```python
from build123d import *

# Parameters (mm, degrees)
SKETCH1_W           = 234
SKETCH1_H           = 75
BOSS_EXTRUDE1_DEPTH = 5.7
SKETCH2_W           = 5.7
SKETCH2_H           = 55
CUT_EXTRUDE1_DEPTH  = 5.7
SKETCH3_W           = 174
SKETCH3_H           = 5.7
CUT_EXTRUDE2_DEPTH  = 5.7
SKETCH4_R           = 1.5
CUT_EXTRUDE3_DEPTH  = 2


with BuildPart() as part:
    # Sketch1 → Boss-Extrude1 (new body)
    with BuildSketch(Plane(origin=(0, 0, 0), x_dir=(1, 0, 0), z_dir=(0, 1, 0))):
        with Locations((117, 37.5)):
            Rectangle(SKETCH1_W, SKETCH1_H)
    extrude(amount=BOSS_EXTRUDE1_DEPTH)

    # Sketch2 → Cut-Extrude1 (cut)
    with BuildSketch(Plane(origin=(0, 5.7, 0), x_dir=(1, 0, 0), z_dir=(0, 1, 0))):
        with Locations((2.85, 37.5)):
            Rectangle(SKETCH2_W, SKETCH2_H)
        with Locations((231.15, 37.5)):
            Rectangle(SKETCH2_W, SKETCH2_H)
    extrude(amount=-CUT_EXTRUDE1_DEPTH, mode=Mode.SUBTRACT)

    # Sketch3 → Cut-Extrude2 (cut)
    with BuildSketch(Plane(origin=(0, 5.7, 0), x_dir=(1, 0, 0), z_dir=(0, 1, 0))):
        with Locations((117, 2.85)):
            Rectangle(SKETCH3_W, SKETCH3_H)
    extrude(amount=-CUT_EXTRUDE2_DEPTH, mode=Mode.SUBTRACT)

    # Sketch4 → Cut-Extrude3 (cut)
    with BuildSketch(Plane(origin=(0, 5.7, 0), x_dir=(1, 0, 0), z_dir=(0, 1, 0))):
        with Locations(Location((213.3, 45.7, 0), (0, 0, 270))):
            Circle(SKETCH4_R)
        with Locations(Location((213.3, 10.7, 0), (0, 0, 270))):
            Circle(SKETCH4_R)
        with Locations(Location((20.7, 10.7, 0), (0, 0, 270))):
            Circle(SKETCH4_R)
        with Locations(Location((20.7, 45.7, 0), (0, 0, 270))):
            Circle(SKETCH4_R)
    extrude(amount=-CUT_EXTRUDE3_DEPTH, mode=Mode.SUBTRACT)


solid = part.part
```
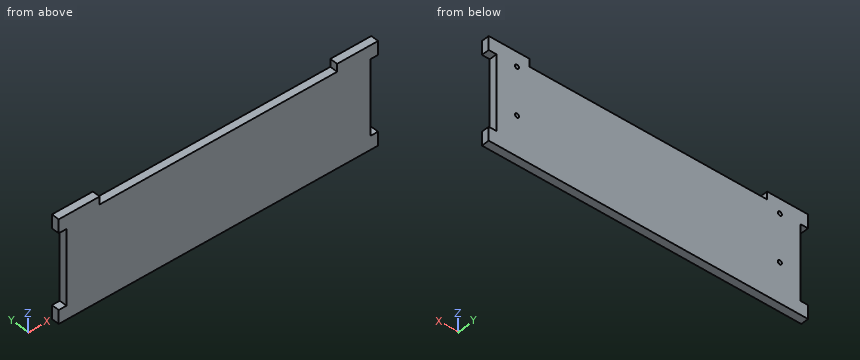
Geometry check sheet. Reference: the model listing, model coordinates, mm. Coordinates: 2 decimals unless noted, no trailing zeros. Write each loop counter-clockwise with the first axis right and the second up, starting at its lowest first coordinate (ties: lowest second). Pieces come first, ordered by that corner, then holes. Notation, with made-up numbers: M 35.5,-30 L 66.5,-30 A18 cw 66.5,-9 Z; hole C -26,69 d6. An arc over 180 degrees is marked long. Answer as a JSON object with one key per item and string values.
1. Section check A-A, the plane y = 2.2. Enter the section's corners in (x, z).
Answers below:
{"outline": "M 0,-75 L 234,-75 L 234,-65 L 228.3,-65 L 228.3,-10 L 234,-10 L 234,0 L 204,0 L 204,-5.7 L 30,-5.7 L 30,0 L 0,0 L 0,-10 L 5.7,-10 L 5.7,-65 L 0,-65 Z"}
2. Section check C-C, the plane z = -35.5. Enter the section's corners in (x, y), plus the area to 3 significant figures.
Answers below:
{"outline": "M 5.7,0 L 228.3,0 L 228.3,5.7 L 5.7,5.7 Z", "area": "1,270 mm²"}
3. Section check B-B, the plane x = 96.5. Enter the section's corners in (y, z), plus the area to 3 significant figures.
Answers below:
{"outline": "M 0,-75 L 5.7,-75 L 5.7,-5.7 L 0,-5.7 Z", "area": "395 mm²"}
4. Go/stop test with flat-tipped pins: pin 1 Ø0.9 at (x, z) = (213, -10.5) entering from +Y; pin 2 Ø2 at (y, z) = (3, -51.5) entering from +X; pin 3 Ø3 at (y, z) = (3, -29.5) entering from -X. Record where each tip stops, or that it passes through.
Answers below:
{"pin 1": "stops at y = 3.7", "pin 2": "stops at x = 228.3", "pin 3": "stops at x = 5.7"}
5. Scan lines: L1, parallel to Z at x = 213.3, y = 4.2; L2, parallel to X at y = 5.15, z = -10.7; L3, parallel to Z at x = 154, y = 4.25. Record each from-to range of solid material in increasing order.
Answers below:
{"L1": "z = -75 to -47.2, -44.2 to -12.2, -9.2 to 0", "L2": "x = 5.7 to 19.2, 22.2 to 211.8, 214.8 to 228.3", "L3": "z = -75 to -5.7"}
